Check sheet for the modelled part. Datum: model origin and axes. Units: mm. A direction names the side the tool comes from. Give positions to 0.01 mm unless a question says otherwise; leave off trailing zeros. Write each loop counter-clockwise with the first axis right and the second up, starting at its lowest first coordinate (ties: lowest second). Pieces come first, ordered by that corner, then holes. Notation, with made-up numbers: (2.25, 88) -> (50.25, 88) arc R5 cw to (50.25, 92) -> close; hole circle Ø1 at (10, 23). An arc over 180 degrees is marked (long way). Return JSON: item names as keys, results as strings.
Autodesk Fusion 360 part; units mm, degrees
sketch "Sketch1" plane through (0, 0, 0) normal (0, 0, 1) x (1, 0, 0)
  line L0 (0, 0) -> (3.4, 0)
  line L1 (3.4, 0) -> (6.8, 5.889)
  line L2 (6.8, 5.889) -> (3.4, 11.7779)
  line L3 (3.4, 11.7779) -> (-3.4, 11.7779)
  line L4 (-3.4, 11.7779) -> (-6.8, 5.889)
  line L5 (-6.8, 5.889) -> (-3.4, 0)
  line L6 (-3.4, 0) -> (3.4, 0)
  point P0 (0, 5.889)
  dimension "d1" = 3.4
  dimension "d2" = 6.8
extrude "Extrude1" add sketch "Sketch1" along normal blind 10
sketch "Sketch2" plane through (0, 0, 10) normal (0, 0, 1) x (-1, 0, 0)
  line L0 (3.4, 0) -> (-3.4, 0)
  line L1 (-3.4, 0) -> (-6.8, -5.889)
  line L2 (-6.8, -5.889) -> (-3.4, -11.7779)
  line L3 (-3.4, -11.7779) -> (3.4, -11.7779)
  line L4 (3.4, -11.7779) -> (6.8, -5.889)
  line L5 (6.8, -5.889) -> (3.4, 0)
  line L6 (-3.4, 0) -> (3.4, -11.7779)
  line L7 (-3.4, 0) -> (0, -5.889)
  line L8 (0, -5.889) -> (-2.05, -2.3383)
  line L9 (-2.05, -2.3383) -> (-4.1, -5.889)
  line L10 (-4.1, -5.889) -> (-2.05, -9.4397)
  line L11 (-2.05, -9.4397) -> (2.05, -9.4397)
  line L12 (2.05, -9.4397) -> (4.1, -5.889)
  line L13 (4.1, -5.889) -> (2.05, -2.3383)
  line L14 (2.05, -2.3383) -> (-2.05, -2.3383)
  line L15 (-2.05, -2.3383) -> (-2.0499, -2.3383) construction
  point P0 (0.025, -5.9323)
  point P1 (0, -5.889)
  dimension "d10" = 6.8
  dimension "d11" = 4.1
  dimension "d12" = 4.1
  dimension "d13" = 0
extrude "Extrude2" add sketch "Sketch2" along normal blind 5 contours L6 L7 L8 L12 L13 L14 | L6 L7 L8 L9 L10 L11
extrude "Extrude3" add 1 faces at (-0.6833, 0.7794, 10) along direction (0, 0, 1) blind 6
extrude "Extrude4" cut 1 faces at (0.6833, 4.7054, 15) along direction (0, 0, -1) blind 10
extrude "Extrude5" cut 1 faces at (-0.6833, 0.7794, 16) along direction (0, 0, -1) blind 1
sketch "Sketch3" plane through (0, 0, 5) normal (0, 0, 1) x (-1, 0, 0)
  line L0 (2.05, -2.3383) -> (-2.05, -2.3383)
  line L1 (-2.05, -2.3383) -> (-4.1, -5.889)
  line L2 (-4.1, -5.889) -> (-2.05, -9.4397)
  line L3 (-2.05, -9.4397) -> (2.05, -9.4397)
  line L4 (2.05, -9.4397) -> (4.1, -5.889)
  line L5 (4.1, -5.889) -> (2.05, -2.3383)
  line L6 (-2.05, -9.4397) -> (0, -5.889)
  circle A0 centre (0, -5.889) radius 1.5
  dimension "d22" = 3
extrude "Extrude6" cut sketch "Sketch3" against normal blind 5 contours A0
sketch "Sketch4" plane through (0, 0, 15) normal (0, 0, 1) x (-1, 0, 0)
  line L0 (2.05, -2.3383) -> (4.1, -5.889)
  line L1 (4.1, -5.889) -> (2.05, -9.4397)
  line L2 (2.05, -9.4397) -> (-2.05, -9.4397)
  line L3 (-2.05, -9.4397) -> (-4.1, -5.889)
  line L4 (-4.1, -5.889) -> (-2.05, -2.3383)
  line L5 (-2.05, -2.3383) -> (2.05, -2.3383)
  line L6 (3.4, 0) -> (-3.4, 0)
  line L7 (-3.4, 0) -> (-6.8, -5.889)
  line L8 (-6.8, -5.889) -> (-3.4, -11.7779)
  line L9 (-3.4, -11.7779) -> (3.4, -11.7779)
  line L10 (3.4, -11.7779) -> (6.8, -5.889)
  line L11 (6.8, -5.889) -> (3.4, 0)
  line L12 (-2.05, -2.3383) -> (2.05, -9.4397)
  line L13 (2.05, -9.4397) -> (0, -5.889)
  line L14 (-2.05, -2.3383) -> (0, -5.889)
  line L15 (0, -5.889) -> (-2.3125, -1.8836)
  line L16 (-2.3125, -1.8836) -> (-4.625, -5.889)
  line L17 (-4.625, -5.889) -> (-2.3125, -9.8943)
  line L18 (-2.3125, -9.8943) -> (2.3125, -9.8943)
  line L19 (2.3125, -9.8943) -> (4.625, -5.889)
  line L20 (4.625, -5.889) -> (2.3125, -1.8836)
  line L21 (2.3125, -1.8836) -> (-2.3125, -1.8836)
  point P0 (0, -5.889)
  dimension "d25" = 4.625
  dimension "d26" = 4.625
extrude "Extrude7" cut sketch "Sketch4" against normal blind 10 contours L16 L17 L18 L19 L20 L21
extrude "Extrude8" cut 1 faces at (0.0374, 1.4644, 0) along direction (0, 0, 1) blind 2
extrude "Extrude9" add 1 faces at (0.7708, 0.6279, 15) along direction (0, 0, 1) blind 2
(1) Cross-section at B-B on z = 8.25. Enter the section's corners in (x, y) (1 decimal), then the cut area to 3 significant figures.
Reply:
{"outline": "(-6.8, 5.9) -> (-3.4, 0) -> (3.4, 0) -> (6.8, 5.9) -> (3.4, 11.8) -> (-3.4, 11.8) -> close; hole (-4.6, 5.9) -> (-2.3, 1.9) -> (2.3, 1.9) -> (4.6, 5.9) -> (2.3, 9.9) -> (-2.3, 9.9) -> close", "area": "64.6 mm^2"}
(2) Cross-section at A-A on x = 0. Enter the section's corners in (y, z).
Reply:
{"outline": "(0, 2) -> (4.39, 2) -> (4.39, 5) -> (1.88, 5) -> (1.88, 17) -> (0, 17) -> close; (7.39, 2) -> (11.78, 2) -> (11.78, 17) -> (9.89, 17) -> (9.89, 5) -> (7.39, 5) -> close"}
(3) Release check for a two-part mould opening along X. For faces 1 (the flat face through (0, 11.778, 9)), 2 (the flat face through (5.124, 8.792, 9.395)), 3 (the flat face through (-2, 6, 5)) record: pulls with the +X half, pulls with the -X half, needs draft (parallel to the pull), parting line crosses it, or undercut.
Reply:
{"face 1": "needs draft", "face 2": "pulls with the +X half", "face 3": "undercut"}
(4) Thickness scan on L1, parallel to Y at x = 0.25, z = 11.25; L2, parallel to Y at x = 0, z = 2.8; L3, parallel to Z at x = -1.75, y = 9. Record the ranges inside material, lowest first.
Reply:
{"L1": "0 to 1.88, 9.89 to 11.78", "L2": "0 to 4.39, 7.39 to 11.78", "L3": "2 to 5"}
(5) Cross-section at D-D on z = 4. Enter the section's corners in (x, y).
Reply:
{"outline": "(-6.8, 5.89) -> (-3.4, 0) -> (3.4, 0) -> (6.8, 5.89) -> (3.4, 11.78) -> (-3.4, 11.78) -> close; hole circle Ø3 at (0, 5.89)"}
(6) Depth check by flat-ended pin: pin 1 Ø5 at (y, z) = (8, 7.5) entering from +X; pin 2 Ø3 at (y, z) = (6, 8.5) entering from -X; pin 3 Ø4 at (x, y) = (0.5, 5) entering from +Z; pin 4 Ø2.5 at (x, y) = (0, 5.889) entering from -Z. Enter the tip coordinate at first touch or a pass-through.
Reply:
{"pin 1": "x = 6.8", "pin 2": "x = -6.8", "pin 3": "z = 5", "pin 4": "through"}
(7) Cross-section at C-C on y = 7. Enter the section's corners in (x, z).
Reply:
{"outline": "(-6.16, 2) -> (-1.01, 2) -> (-1.01, 5) -> (-3.98, 5) -> (-3.98, 17) -> (-6.16, 17) -> close; (1.01, 2) -> (6.16, 2) -> (6.16, 17) -> (3.98, 17) -> (3.98, 5) -> (1.01, 5) -> close"}
(8) Set-up check for faces 4 (the flat face through (5.076, 2.903, 9.395)), 5 (the flat face through (0, 9.894, 11)): record each of +Z, -Z, +X, -X, +Y, -Y from which the full face is reachable in a straight line by a thin tool's end or side.
Reply:
{"face 4": "+Z, -Z, +X, -Y", "face 5": "+Z"}
